The model under review builds one solid part; all positions refer to its coordinate system, in mm. Give positions to 0.01 mm unless a question says otherwise; leave off trailing zeros. Write each loop counter-clockwise with the first axis right and the second up, starting at its lowest first coordinate (ties: lowest second). Pieces come first, ordered by that corner, then holes. Notation, with made-up numbers: M 43.5,49 L 93.5,49 A12 ccw 93.5,64 Z; hole C 3.5,16 d3. An arc over 180 degrees is marked long. Write each question's results on one line, items separated by ' | '. Start each with the question number.
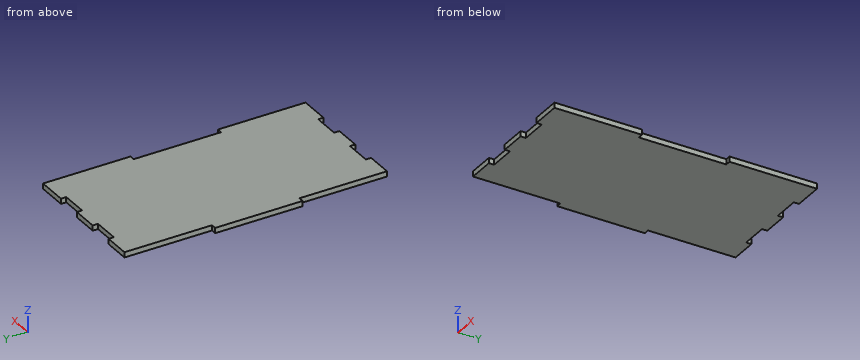
Autodesk Inventor part; units mm, degrees
ref_plane "YZ Plane" through (0, 0, 0) normal (1, 0, 0) x (0, 1, 0)
ref_plane "XZ Plane" through (0, 0, 0) normal (0, 1, 0) x (-1, 0, 0)
ref_plane "XY Plane" through (0, 0, 0) normal (0, 0, 1) x (1, 0, 0)
sketch "Boceto1" plane through (0, 0, 0) normal (0, 0, 1) x (1, 0, 0)
  line L0 (0, 0) -> (80, 0)
  line L1 (80, 0) -> (80, 150)
  line L2 (80, 150) -> (0, 150)
  line L3 (0, 150) -> (0, 0)
  dimension "d0" = 80
  dimension "d1" = 150
extrude "Extrusión1" add sketch "Boceto1" along normal blind 3
sketch "Boceto2" plane through (0, 0, 3) normal (0, 0, 1) x (1, 0, 0)
  line L0 (0, 0) -> (80, 0) construction
  line L1 (80, 0) -> (80, 150) construction
  line L2 (80, 150) -> (0, 150) construction
  line L3 (0, 150) -> (0, 0) construction
  line L4 (3, 0) -> (0, 0)
  line L5 (0, 0) -> (0, 50)
  line L6 (0, 50) -> (3, 50)
  line L7 (3, 50) -> (3, 0)
  line L8 (0, 150) -> (3, 150)
  line L9 (3, 150) -> (3, 100)
  line L10 (3, 100) -> (0, 100)
  line L11 (0, 100) -> (0, 150)
  line L12 (77, 100) -> (80, 100)
  line L13 (80, 100) -> (80, 50)
  line L14 (80, 50) -> (77, 50)
  line L15 (77, 50) -> (77, 100)
  line L16 (80, 0) -> (80, 150) construction
  point P0 (80, 75)
  point P1 (80, 75)
  dimension "d4" = 3
  dimension "d5" = 50
  dimension "d6" = 3
  dimension "d7" = 50
  dimension "d8" = 50
  dimension "d9" = 3
extrude "Extrusión2" cut sketch "Boceto2" against normal blind 3
sketch "Boceto3" plane through (0, 0, 3) normal (0, 0, 1) x (1, 0, 0)
  line L0 (3, 50) -> (3, 0) construction
  line L1 (3, 0) -> (80, 0) construction
  line L2 (80, 0) -> (80, 50) construction
  line L3 (80, 50) -> (77, 50) construction
  line L4 (77, 50) -> (77, 100) construction
  line L5 (77, 100) -> (80, 100) construction
  line L6 (80, 100) -> (80, 150) construction
  line L7 (80, 150) -> (3, 150) construction
  line L8 (3, 150) -> (3, 100) construction
  line L9 (3, 100) -> (0, 100) construction
  line L10 (0, 100) -> (0, 50) construction
  line L11 (0, 50) -> (3, 50) construction
  line L12 (18, 3) -> (33, 3)
  line L13 (33, 3) -> (33, 0)
  line L14 (33, 0) -> (18, 0)
  line L15 (18, 0) -> (18, 3)
  line L16 (48, 3) -> (63, 3)
  line L17 (63, 3) -> (63, 0)
  line L18 (63, 0) -> (48, 0)
  line L19 (48, 0) -> (48, 3)
  line L20 (3, 0) -> (80, 0) construction
  line L21 (18, 150) -> (33, 150)
  line L22 (33, 150) -> (33, 147)
  line L23 (33, 147) -> (18, 147)
  line L24 (18, 147) -> (18, 150)
  line L25 (48, 147) -> (63, 147)
  line L26 (63, 147) -> (63, 150)
  line L27 (63, 150) -> (48, 150)
  line L28 (48, 150) -> (48, 147)
  line L29 (80, 150) -> (3, 150) construction
  point P0 (0, 0)
  dimension "d12" = 3
  dimension "d13" = 15
  dimension "d14" = 15
  dimension "d15" = 3
  dimension "d16" = 15
  dimension "d17" = 15
  dimension "d20" = 3
  dimension "d21" = 3
  dimension "d22" = 15
  dimension "d23" = 15
  dimension "d24" = 15
  dimension "d25" = 15
extrude "Extrusión3" cut sketch "Boceto3" against normal blind 10 contours L12 L13 L14 L15 | L16 L17 L18 L19
sketch "Boceto4" plane through (0, 0, 3) normal (0, 0, 1) x (1, 0, 0)
  line L0 (33, 3) -> (33, 0) construction
  line L1 (33, 0) -> (48, 0) construction
  line L2 (48, 0) -> (48, 3) construction
  line L3 (48, 3) -> (63, 3) construction
  line L4 (63, 3) -> (63, 0) construction
  line L5 (63, 0) -> (80, 0) construction
  line L6 (80, 0) -> (80, 50) construction
  line L7 (80, 50) -> (77, 50) construction
  line L8 (77, 50) -> (77, 100) construction
  line L9 (77, 100) -> (80, 100) construction
  line L10 (80, 100) -> (80, 150) construction
  line L11 (80, 150) -> (3, 150) construction
  line L12 (3, 150) -> (3, 100) construction
  line L13 (3, 100) -> (0, 100) construction
  line L14 (0, 100) -> (0, 50) construction
  line L15 (0, 50) -> (3, 50) construction
  line L16 (3, 50) -> (3, 0) construction
  line L17 (3, 0) -> (18, 0) construction
  line L18 (18, 0) -> (18, 3) construction
  line L19 (18, 3) -> (33, 3) construction
  line L20 (18, 150) -> (33, 150)
  line L21 (33, 150) -> (33, 147)
  line L22 (33, 147) -> (18, 147)
  line L23 (18, 147) -> (18, 150)
  line L24 (48, 150) -> (63, 150)
  line L25 (63, 150) -> (63, 147)
  line L26 (63, 147) -> (48, 147)
  line L27 (48, 147) -> (48, 150)
  line L28 (80, 150) -> (3, 150) construction
  point P0 (0, 0)
  dimension "d26" = 15
  dimension "d27" = 15
  dimension "d28" = 15
  dimension "d29" = 15
  dimension "d30" = 3
extrude "Extrusión4" cut sketch "Boceto4" against normal blind 10
equation "\"d6\" = d4"
equation "\"d7\" = d5"
equation "\"d8\" = d7"
equation "\"d9\" = d4"
properties part number "Pared Garita"
(1) Clearance check with flat-ended pins moving along their axes: P1, Ø0.9, axis at y = 68, z = 2, coming from the +X side; P2, Ø0.9, axis at x = 1, z = 1.5, coming from the +Y side; P3, Ø1.5, axis at y = 1.5, z = 1.5, coming from the -X side. State where each tip first meets the part, or that it passes through.
(2) Add section B-B (y = 92). State the section outline as (x, z) points.
(3) Wall thickness on L1, parallel to Y at x = 19.5, z = 1.15; L2, parallel to X at y = 78.5, z = 1.45; L3, parallel to X at y = 130, z = 2.45: over which ranges is each line inside the solid? List them lowest first.
(4) Add section A-A (z = 1). State the section outline as (x, y) points, then the cut area to 3 significant figures.
(5) Add section C-C (x = 20.5). State the section outline as (y, z) points.
Calculated:
1) P1: stops at x = 77 | P2: stops at y = 100 | P3: stops at x = 3
2) outline: M 0,0 L 77,0 L 77,3 L 0,3 Z
3) L1: y = 3 to 147 | L2: x = 0 to 77 | L3: x = 3 to 80
4) outline: M 0,50 L 3,50 L 3,0 L 18,0 L 18,3 L 33,3 L 33,0 L 48,0 L 48,3 L 63,3 L 63,0 L 80,0 L 80,50 L 77,50 L 77,100 L 80,100 L 80,150 L 63,150 L 63,147 L 48,147 L 48,150 L 33,150 L 33,147 L 18,147 L 18,150 L 3,150 L 3,100 L 0,100 Z | area: 11,400 mm²
5) outline: M 3,0 L 147,0 L 147,3 L 3,3 Z
